from build123d import *

# Parameters (mm, degrees)
SKETCH1_W           = 50.8
SKETCH1_H           = 40
SKETCH1_R           = 8
BOSS_EXTRUDE1_DEPTH = 6
FILLET1_R           = 6.35
SKETCH8_R           = 1.5
CUT_EXTRUDE1_DEPTH  = 33.880997552
SKETCH9_R           = 1.8
M3_THROUGH_DEPTH    = 33.880997552
MOVE_FACE2_BY       = 0.1
MOVE_FACE2_2_BY     = 0.1
MOVE_FACE2_3_BY     = 0.1
MOVE_FACE2_4_BY     = 0.1
MOVE_FACE2_5_BY     = 0.1
MOVE_FACE2_6_BY     = 0.1
MOVE_FACE2_7_BY     = 0.1
MOVE_FACE2_8_BY     = 0.1
MOVE_FACE2_9_BY     = 0.1
MOVE_FACE2_10_BY    = 0.1
MOVE_FACE2_11_BY    = 0.1
MOVE_FACE2_12_BY    = 0.1
MOVE_FACE2_13_BY    = 0.1
MOVE_FACE2_14_BY    = 0.1
MOVE_FACE2_15_BY    = 0.1
MOVE_FACE2_16_BY    = 0.1
MOVE_FACE2_17_BY    = 0.1
MOVE_FACE2_18_BY    = 0.1
MOVE_FACE2_19_BY    = 0.1
MOVE_FACE2_20_BY    = 0.1
MOVE_FACE2_21_BY    = 0.1


with BuildPart() as part:
    # Sketch1 → Boss-Extrude1 (new body)
    with BuildSketch(Plane.XY):
        Rectangle(SKETCH1_W, SKETCH1_H)
        Circle(SKETCH1_R, mode=Mode.SUBTRACT)
    extrude(amount=BOSS_EXTRUDE1_DEPTH)

    # Fillet1
    fillet1_edges = [part.edges().sort_by_distance(p)[0] for p in [
        (-25.4, 20, 3),
        (25.4, 20, 3),
        (25.4, -20, 3),
        (-25.4, -20, 3),
    ]]
    fillet(fillet1_edges, radius=FILLET1_R)

    # Sketch8 → Cut-Extrude1 (cut, through all)
    with BuildSketch(Plane.XY.offset(6)):
        with Locations((22.225, 0)):
            Circle(SKETCH8_R)
        with Locations((-22.225, 0)):
            Circle(SKETCH8_R)
    extrude(amount=-CUT_EXTRUDE1_DEPTH, mode=Mode.SUBTRACT)

    # Sketch9 → M3-through (cut, through all)
    with BuildSketch(Plane.XY.offset(6)):
        with Locations((-19.05, 13.65)):
            Circle(SKETCH9_R)
        with Locations(Location((-19.05, -13.65, 0), (0, 0, 180))):
            Circle(SKETCH9_R)
        with Locations((19.05, -13.65)):
            Circle(SKETCH9_R)
        with Locations(Location((19.05, 13.65, 0), (0, 0, 180))):
            Circle(SKETCH9_R)
        with Locations((11, 0)):
            Circle(SKETCH9_R)
        with Locations((5.5, -9.526279442)):
            Circle(SKETCH9_R)
        with Locations((-5.5, -9.526279442)):
            Circle(SKETCH9_R)
        with Locations((-11, 0)):
            Circle(SKETCH9_R)
        with Locations((-5.5, 9.526279442)):
            Circle(SKETCH9_R)
        with Locations((5.5, 9.526279442)):
            Circle(SKETCH9_R)
    extrude(amount=-M3_THROUGH_DEPTH, mode=Mode.SUBTRACT)

    # Move Face2: a face moved outward by 0.1
    extrude(part.faces().sort_by_distance((-25.4, 0, 3))[0], amount=MOVE_FACE2_BY, dir=(-1, 0, 0))

    # Move Face2 2: a curved face moved outward by 0.1
    add(Solid.thicken(part.faces().sort_by_distance((-23.540128061, 18.140128061, 3))[0], MOVE_FACE2_2_BY))

    # Move Face2 3: a face moved outward by 0.1
    extrude(part.faces().sort_by_distance((0, 20, 3))[0], amount=MOVE_FACE2_3_BY, dir=(0, 1, 0))

    # Move Face2 4: a curved face moved outward by 0.1
    add(Solid.thicken(part.faces().sort_by_distance((23.540128061, 18.140128061, 3))[0], MOVE_FACE2_4_BY))

    # Move Face2 5: a face moved outward by 0.1
    extrude(part.faces().sort_by_distance((25.4, 0, 3))[0], amount=MOVE_FACE2_5_BY, dir=(1, 0, 0))

    # Move Face2 6: a face moved outward by 0.1
    extrude(part.faces().sort_by_distance((0, -20, 3))[0], amount=MOVE_FACE2_6_BY, dir=(0, -1, 0))

    # Move Face2 7: a curved face moved outward by 0.1
    add(Solid.thicken(part.faces().sort_by_distance((-17.25, -13.65, 3))[0], MOVE_FACE2_7_BY))

    # Move Face2 8: a curved face moved outward by 0.1
    add(Solid.thicken(part.faces().sort_by_distance((-8, 0, 3))[0], MOVE_FACE2_8_BY))

    # Move Face2 9: a curved face moved outward by 0.1
    add(Solid.thicken(part.faces().sort_by_distance((20.725, 0, 3))[0], MOVE_FACE2_9_BY))

    # Move Face2 10: a curved face moved outward by 0.1
    add(Solid.thicken(part.faces().sort_by_distance((-23.725, 0, 3))[0], MOVE_FACE2_10_BY))

    # Move Face2 11: a curved face moved outward by 0.1
    add(Solid.thicken(part.faces().sort_by_distance((-20.85, 13.65, 3))[0], MOVE_FACE2_11_BY))

    # Move Face2 12: a curved face moved outward by 0.1
    add(Solid.thicken(part.faces().sort_by_distance((17.25, -13.65, 3))[0], MOVE_FACE2_12_BY))

    # Move Face2 13: a curved face moved outward by 0.1
    add(Solid.thicken(part.faces().sort_by_distance((20.85, 13.65, 3))[0], MOVE_FACE2_13_BY))

    # Move Face2 14: a curved face moved outward by 0.1
    add(Solid.thicken(part.faces().sort_by_distance((9.2, 0, 3))[0], MOVE_FACE2_14_BY))

    # Move Face2 15: a curved face moved outward by 0.1
    add(Solid.thicken(part.faces().sort_by_distance((3.7, -9.526279442, 3))[0], MOVE_FACE2_15_BY))

    # Move Face2 16: a curved face moved outward by 0.1
    add(Solid.thicken(part.faces().sort_by_distance((-7.3, -9.526279442, 3))[0], MOVE_FACE2_16_BY))

    # Move Face2 17: a curved face moved outward by 0.1
    add(Solid.thicken(part.faces().sort_by_distance((-12.8, 0, 3))[0], MOVE_FACE2_17_BY))

    # Move Face2 18: a curved face moved outward by 0.1
    add(Solid.thicken(part.faces().sort_by_distance((-7.3, 9.526279442, 3))[0], MOVE_FACE2_18_BY))

    # Move Face2 19: a curved face moved outward by 0.1
    add(Solid.thicken(part.faces().sort_by_distance((3.7, 9.526279442, 3))[0], MOVE_FACE2_19_BY))

    # Move Face2 20: a curved face moved outward by 0.1
    add(Solid.thicken(part.faces().sort_by_distance((-23.540128061, -18.140128061, 3))[0], MOVE_FACE2_20_BY))

    # Move Face2 21: a curved face moved outward by 0.1
    add(Solid.thicken(part.faces().sort_by_distance((23.540128061, -18.140128061, 3))[0], MOVE_FACE2_21_BY))


solid = part.part
Model file for the job. Use its own axes, mm. Give positions to 0.01 mm unless a question says otherwise; leave off trailing zeros. Loops run counter-clockwise (first coordinate to the right, second up) from the corner with the lowest first, then second, coordinate; pieces in that order, holes last.
1) Saw through at C-C (y = -10.5). Write the cut outline in (x, z), plus the area to 3 significant figures.
2) Saw through at B-B (x = -5.5). Write the cut outline in (y, z).
3) Flat gauge pin, fed straight in: pin 1 Ø1 at (x, y) = (-13, -1) entering from -Z. Where does the tip first touch, or does it go through?
4) Wall check: line 1 (Y direction, x = -19.05, z = 3.4); line 2 (Y direction, x = 20, z = 5.7); line 3 (X direction, y = 13, z = 5.5). Give the ranges that are in metal, low to high.
5) Pull direction X, two halves, no side cores. Call faces 1 (the flat face through (0, -9, 0)), 2 (the cylindrical face through (18.27, 15.16, 3.04)), 3 (the flat face through (25.5, 0, 3)): +X half, -X half, draft (parallel to the pull), parting line (faces both ways), or undercut.
6) Saw through at D-D (z = 1.3). Count the separate pieces of the cut face and the enclosed holes in it, plus the area to 3 significant figures.
7) Saw through at A-A (y = 5). Write the cut outline in (x, z), plus the area to 3 significant figures.
Answer block:
1. outline: (-25.5, 0) - (-6.89, 0) - (-6.89, 6) - (-25.5, 6) - close; (-4.11, 0) - (4.11, 0) - (4.11, 6) - (-4.11, 6) - close; (6.89, 0) - (25.5, 0) - (25.5, 6) - (6.89, 6) - close
1. area: 273 mm2
2. outline: (-20.1, 0) - (-11.23, 0) - (-11.23, 6) - (-20.1, 6) - close; (-7.83, 0) - (-5.67, 0) - (-5.67, 6) - (-7.83, 6) - close; (5.67, 0) - (7.83, 0) - (7.83, 6) - (5.67, 6) - close; (11.23, 0) - (20.1, 0) - (20.1, 6) - (11.23, 6) - close
3. pin 1: stops at z = 0
4. line 1: y = -20.1 to -15.35, -11.95 to 11.95, 15.35 to 20.1
4. line 2: y = -20.03 to -15.06, -12.24 to 12.24, 15.06 to 20.03
4. line 3: x = -25.5 to -20.62, -17.48 to 17.48, 20.62 to 25.5
5. face 1: draft
5. face 2: undercut
5. face 3: +X half
6. separate pieces: 1
6. enclosed holes: 13
6. area: 1,720 mm2
7. outline: (-25.5, 0) - (-6.12, 0) - (-6.12, 6) - (-25.5, 6) - close; (6.12, 0) - (25.5, 0) - (25.5, 6) - (6.12, 6) - close
7. area: 233 mm2
